CAD build for the part. Positions are in the model's coordinates, mm. Face numbers are marked on the shaded views. A direction names the side the tool comes from. Round coordinates to 2 decimals unless told otherwise and drop trailing zeros. Loops run counter-clockwise (first coordinate to the right, second up) from the corner with the lowest first, then second, coordinate; pieces in that order, holes last. Notation, with made-up numbers: M 59,6.5 L 95,6.5 A17 ccw 95,26.5 Z; hole C -17,69 d4. An arc over 180 degrees is marked long. Use one line per item in the form item = value.
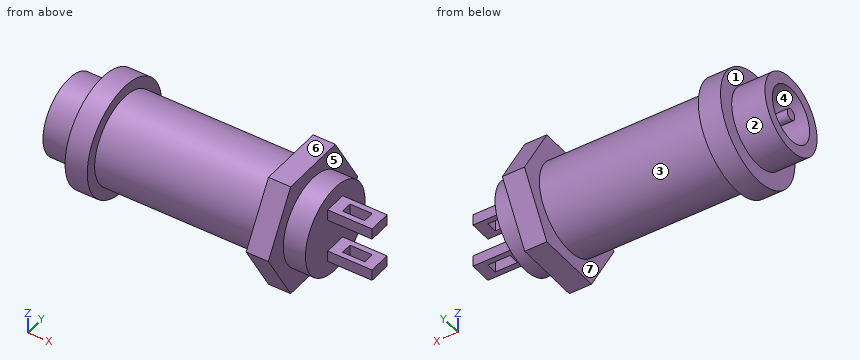
from build123d import *

# Parameters (mm, degrees)
CORTAR_EXTRUIR2_DEPTH   = 2
CROQUIS3_W              = 1
CROQUIS3_H              = 2
SALIENTE_EXTRUIR1_DEPTH = 4
CROQUIS5_W              = 2
CROQUIS5_H              = 1
CORTAR_EXTRUIR3_DEPTH   = 10


with BuildPart() as part:
    # Croquis1 → Revolución1 (revolve)
    with BuildSketch(Plane.XY):
        Polygon((0, 0), (0, 0.5), (10, 0.5), (10, 2.5), (0, 2.5), (0, 3.5), (3, 3.5), (3, 5), (5, 5), (5, 4), (20, 4), (20, 6), (22, 6), (22, 4), (24, 4), (24, 0), align=None)
    revolve(axis=Axis((24, 0, 0), (-1, 0, 0)))

    # Croquis2 → Cortar-Extruir2 (cut)
    with BuildSketch(Plane(origin=(22, 0, 0), x_dir=(0, 0, -1), z_dir=(1, 0, 0))):
        with BuildLine():
            ThreePointArc((5.196152423, 3), (3, 5.196152423), (0, 6))
            Line((0, 6), (5.196152423, 3))
        make_face()
        with BuildLine():
            Line((-5.196152423, 3), (0, 6))
            ThreePointArc((0, 6), (-3, 5.196152423), (-5.196152423, 3))
        make_face()
        with BuildLine():
            Line((-5.196152423, -3), (-5.196152423, 3))
            ThreePointArc((-5.196152423, 3), (-6, 0), (-5.196152423, -3))
        make_face()
        with BuildLine():
            ThreePointArc((5.196152423, -3), (6, 0), (5.196152423, 3))
            Line((5.196152423, 3), (5.196152423, -3))
        make_face()
        with BuildLine():
            Line((0, -6), (-5.196152423, -3))
            ThreePointArc((-5.196152423, -3), (-3, -5.196152423), (0, -6))
        make_face()
        with BuildLine():
            ThreePointArc((0, -6), (3, -5.196152423), (5.196152423, -3))
            Line((5.196152423, -3), (0, -6))
        make_face()
    extrude(amount=-CORTAR_EXTRUIR2_DEPTH, mode=Mode.SUBTRACT)

    # Croquis3 → Saliente-Extruir1 (add)
    with BuildSketch(Plane(origin=(24, 0, 0), x_dir=(0, 0, -1), z_dir=(1, 0, 0))):
        with Locations((-2, -0.001163142)):
            Rectangle(CROQUIS3_W, CROQUIS3_H)
        with Locations((2, 0)):
            Rectangle(CROQUIS3_W, CROQUIS3_H)
    extrude(amount=SALIENTE_EXTRUIR1_DEPTH)

    # Croquis5 → Cortar-Extruir3 (cut)
    with BuildSketch(Plane(origin=(0, 0, -2.5), x_dir=(-1, 0, 0), z_dir=(0, 0, -1))):
        with Locations((-26, 0)):
            Rectangle(CROQUIS5_W, CROQUIS5_H)
    extrude(amount=-CORTAR_EXTRUIR3_DEPTH, mode=Mode.SUBTRACT)


solid = part.part
1. Tool access for the marked faces 4, 5, 6 and 7: list every direction of +Z, -Z, +X, -X, +Y, -Y with a clear straight run to the whole face (end or side of a thin tool).
Completed:
face_4 = -X
face_5 = +X
face_6 = +Z, +X, -X, +Y, -Y
face_7 = none
2. Cut at D-D on x = 15. Write the cut outline in (y, z), and give its area (3 significant figures).
Completed:
outline = C 0,0 d8
area = 50.3 mm2
3. Pull direction X, two halves, no side cores. Call the marked faces 1, 2 and 3: +X half, -X half, draft (parallel to the pull), parting line (faces both ways), or undercut.
Completed:
face_1 = -X half
face_2 = draft
face_3 = undercut
4. Cut at A-A on x = 3.5. Write the cut outline in (y, z), and give its area (3 significant figures).
Completed:
outline = C 0,0 d10; C 0,0 d1; hole C 0,0 d5
area = 59.7 mm2
5. Probe line 1 along Y through (x, z) = (7.75, 0); line 2 along Y through (x, z) = (4.5, 0). List the from-to ranges inside material, lowest first. Write a range as from..to.
Completed:
line_1 = -4..-2.5, -0.5..0.5, 2.5..4
line_2 = -5..-2.5, -0.5..0.5, 2.5..5
6. Drop flat-ended pins along their axis: P1, Ø0.5, axis at x = 26.5, z = -2, coming from the +Y side; P2, Ø0.6, axis at x = 26.5, y = 0, coming from the -Z side; P3, Ø1, axis at x = 11.5, z = -3, coming from the +Y side; P4, Ø1, axis at y = -3.5, z = 1, coming from the -X side. Give the stop position or say it passes through.
Completed:
P1 = 1
P2 = through
P3 = 3.12
P4 = 0
7. Cut at B-B on y = -4.5. Write the cut outline in (x, z), and give its area (3 significant figures).
Completed:
outline = M 3,-2.18 L 5,-2.18 L 5,2.18 L 3,2.18 Z; M 20,-2.6 L 22,-2.6 L 22,2.6 L 20,2.6 Z
area = 19.1 mm2
